Part model, mm, in its own coordinate system. A direction names the side the tool comes from. Give positions to 0.01 mm unless a question says otherwise; leave off trailing zeros. Write each loop counter-clockwise with the first axis right and the second up, starting at its lowest first coordinate (ties: lowest second). Pieces come first, ordered by that corner, then holes. Notation, with made-up numbers: M 64,71.5 L 89,71.5 A28 ccw 89,108.5 Z; hole C 89,27 d9. An arc over 180 degrees is marked long. Answer as CSV lines item,"result". Start each with the question number.
Item 1: Band-saw the part on A-A, the plane z = -46. List the corners of the cut face in (x, y).
Item 2: Wall check: L1, parallel to X at y = 5, z = -35; L2, parallel to X at y = 1.5, z = -44; L3, parallel to X at y = 2.5, z = 23.5. Give the ranges that are in metal, low to high. Write a range as from..to.
Item 3: Two-plate mould, pull along Y, no slides. Class faces 4 (the flat face through (9, 0.9, 64)), 5 (the flat face through (0, 10, 10)), 6 (the flat face through (0, 2, 59)), 7 (the flat face through (20.5, 6, 28)): +Y half, -Y half, draft (parallel to the pull), parting line (faces both ways), or undercut.
Item 4: 3-axis set-ups, long thin cutter, end or side, ignore diameter. For faces 1 (the flat face through (-26, 5, 35)), 2 (the flat face through (12.5, 5, 31)), 3 (the flat face through (-20.5, 6, 28)): which of +Z, -Z, +X, -X, +Y, -Y reach the whole face in a straight line?
Item 5: Pin check, flat tips, straight feed: pin 1 (4 mm diameter, centred on x = -16, z = 18, fed in from +Y); pin 2 (5 mm diameter, centred on y = 3.5, z = -34, fed in from +X); pin 3 (1.2 mm diameter, centred on x = -0.5, y = 1, fed in from +Z); pin 4 (5 mm diameter, centred on x = 25.5, y = 5, fed in from +Z). Stop position of each tip, or through.
Item 6: Band-saw the part on D-D, the plane z = 18. List the corners of the cut face in (x, y).
Item 7: Band-saw the part on C-C, the plane z = 30.5. List the corners of the cut face in (x, y), then the cut area to 3 significant figures.
Item 8: Band-saw the part on B-B, the plane x = -6. List the corners of the cut face in (y, z).
from build123d import *
from OCP.BRepFilletAPI import BRepFilletAPI_MakeChamfer

# Parameters (mm, degrees)
SKETCH1_W               = 24
SKETCH1_H               = 40
BOSS_EXTRUDE1_DEPTH     = 10
SKETCH2_R               = 7.5
BOSS_EXTRUDE2_DEPTH     = 10
SKETCH4_W               = 2
SKETCH4_H               = 20
SKETCH4_H_2             = 16
CUT_EXTRUDE1_DEPTH      = 20
SKETCH5_R               = 2.4
CUT_EXTRUDE2_DEPTH      = 74
CHAMFER3_SIZE           = 2
CHAMFER3_SIZE2          = 4.613601474
BOSS_EXTRUDE3_DEPTH     = 10
CUT_EXTRUDE3_DEPTH      = 10
CUT_EXTRUDE3_DEPTH_BACK = 10
FILLET1_R               = 10
SKETCH8_W               = 5
SKETCH8_H               = 3
CUT_EXTRUDE4_DEPTH      = 5


with BuildPart() as part:
    # Sketch1 → Boss-Extrude1 (new body)
    with BuildSketch(Plane(origin=(0, 0, 0), x_dir=(1, 0, 0), z_dir=(0, 1, 0))):
        Rectangle(SKETCH1_W, SKETCH1_H)
    extrude(amount=BOSS_EXTRUDE1_DEPTH)

    # Sketch2 → Boss-Extrude2 (add)
    with BuildSketch(Plane.XZ):
        Polygon((7, -20), (-7, -20), (-7, 35), (-32, 35), (-32, -15), (-12.5, -25), (-12.5, -50), (12.5, -50), (12.5, -25), (32, -15), (32, 35), (7, 35), align=None)
        with Locations(Location((0, -35, 0), (0, 0, 270))):
            Circle(SKETCH2_R, mode=Mode.SUBTRACT)
        with Locations(Location((-19.5, 18, 0), (0, 0, 270))):
            Circle(SKETCH2_R, mode=Mode.SUBTRACT)
        with Locations(Location((19.5, 18, 0), (0, 0, 270))):
            Circle(SKETCH2_R, mode=Mode.SUBTRACT)
    extrude(amount=-BOSS_EXTRUDE2_DEPTH)

    # Sketch4 → Cut-Extrude1 (cut)
    with BuildSketch(Plane(origin=(0, 10, 0), x_dir=(1, 0, 0), z_dir=(0, 1, 0))):
        with Locations((19.5, -35)):
            Rectangle(SKETCH4_W, SKETCH4_H)
        with Locations((-19.5, -35)):
            Rectangle(SKETCH4_W, SKETCH4_H)
        with Locations((0, 50)):
            Rectangle(SKETCH4_W, SKETCH4_H_2)
    extrude(amount=-CUT_EXTRUDE1_DEPTH, mode=Mode.SUBTRACT)

    # Sketch5 → Cut-Extrude2 (cut)
    with BuildSketch(Plane(origin=(32, 0, 0), x_dir=(0, 0, -1), z_dir=(1, 0, 0))):
        with Locations(Location((-30.5, 5, 0), (0, 0, 180))):
            Circle(SKETCH5_R)
        with Locations(Location((46, 5, 0), (0, 0, 180))):
            Circle(SKETCH5_R)
    extrude(amount=-CUT_EXTRUDE2_DEPTH, mode=Mode.SUBTRACT)

    # Chamfer3: one chamfer whose edges measure the first distance from different faces: ONE call of the kernel's chamfer builder (chamfer() names one face for all edges)
    chamfer3_edges_1 = [part.edges().sort_by_distance(p)[0] for p in [
        (-12.5, 5, -25),
        (-32, 5, -15),
    ]]
    chamfer3_side_1 = [part.faces().sort_by_distance(p)[0] for p in [
        (-22.25, 5, -20),
    ]]
    chamfer3_edges_2 = [part.edges().sort_by_distance(p)[0] for p in [
        (32, 5, -15),
        (12.5, 5, -25),
    ]]
    chamfer3_side_2 = [part.faces().sort_by_distance(p)[0] for p in [
        (22.25, 5, -20),
    ]]
    chamfer3 = BRepFilletAPI_MakeChamfer(part.part.solid().wrapped)
    for e in chamfer3_edges_1:
        chamfer3.Add(CHAMFER3_SIZE, CHAMFER3_SIZE2, e.wrapped, chamfer3_side_1[0].wrapped)  # the first distance lies on this face
    for e in chamfer3_edges_2:
        chamfer3.Add(CHAMFER3_SIZE, CHAMFER3_SIZE2, e.wrapped, chamfer3_side_2[0].wrapped)  # the first distance lies on this face
    add(Compound.cast(chamfer3.Shape()), mode=Mode.REPLACE)

    # Sketch6 → Boss-Extrude3 (add)
    with BuildSketch(Plane.XZ):
        Polygon((-12.5, 22.639119403), (-12.5, 69), (12.5, 69), (12.5, 22.639119403), (7, 20), (-7, 20), align=None)
    extrude(amount=-BOSS_EXTRUDE3_DEPTH)

    # Sketch7 → Cut-Extrude3 (cut, two sides: drawn at the far end of the back side and taken through both)
    with BuildSketch(Plane.XY.offset(69).offset(-CUT_EXTRUDE3_DEPTH_BACK)):
        Polygon((-10.05, 0.9), (-7.5, 0.9), (-7.5, -1.2), (7.5, -1.2), (7.5, 0.9), (10.05, 0.9), (10.05, 3), (-10.05, 3), align=None)
    extrude(amount=CUT_EXTRUDE3_DEPTH + CUT_EXTRUDE3_DEPTH_BACK, mode=Mode.SUBTRACT)

    # Fillet1
    # the kernel refuses this fillet: 10 mm, written as the material it adds along each edge
    with BuildSketch(Plane(origin=(12.5, 0, -29.613601474), x_dir=(0.3065313660894553, 0, 0.9518605578567336), z_dir=(0, 1, 0)), Plane(origin=(-12.5, 0, -29.613601474), x_dir=(0, 0, -1), z_dir=(0, 1, 0))) as fillet1_piece_1:
        with BuildLine():
            CenterArc((FILLET1_R * 0.15704572996, FILLET1_R), FILLET1_R, 252.149681698, 17.850318302)
            Line((-FILLET1_R * 0.149485636129, FILLET1_R * 0.0481394421433), (0, 0))
            Line((0, 0), (FILLET1_R * 0.15704572996, 0))
        make_face()
    extrude(amount=10)
    with BuildSketch(Plane(origin=(14.279634926, 0, -24.087366705), x_dir=(0.8898174628127374, 0, 0.4563166475962744), z_dir=(0, 1, 0)), Plane(origin=(-14.279634926, 0, -24.087366705), x_dir=(0.30653136608945597, 0, -0.9518605578567335), z_dir=(0, 1, 0))) as fillet1_piece_2:
        with BuildLine():
            CenterArc((FILLET1_R * 0.414213562373, FILLET1_R), FILLET1_R, 225, 45)
            Line((-FILLET1_R * 0.292893218813, FILLET1_R * 0.292893218813), (0, 0))
            Line((0, 0), (FILLET1_R * 0.414213562373, 0))
        make_face()
    extrude(amount=10)
    with BuildSketch(Plane(origin=(12.5, 10, 35), x_dir=(0, 0, 1), z_dir=(0, -1, 0))) as fillet1_piece_3:
        with BuildLine():
            CenterArc((9.16515139, -10), FILLET1_R, 90, 66.421821522)
            Line((0, -6), (0, 0))
            Line((0, 0), (9.16515139, 0))
        make_face()
    extrude(amount=10)
    with BuildSketch(Plane(origin=(-12.5, 0, 35), x_dir=(-1, 0, 0), z_dir=(0, 1, 0))) as fillet1_piece_4:
        with BuildLine():
            CenterArc((10, 9.16515139), FILLET1_R, 180, 66.421821522)
            Line((0, 9.16515139), (0, 0))
            Line((0, 0), (6, 0))
        make_face()
    extrude(amount=10)
    # the kernel refuses this fillet: 10 mm, written as the material it takes off along each edge
    with BuildSketch(Plane(origin=(30.220365074, -10.355339059, -15.912633295), x_dir=(-0.8898174628127375, 0, -0.45631664759627466), z_dir=(0, 1, 0))) as fillet1_2_piece_1:
        with BuildLine():
            CenterArc((FILLET1_R * 0.414213562373, FILLET1_R), FILLET1_R, 225, 45)
            Line((-FILLET1_R * 0.292893218813, FILLET1_R * 0.292893218813), (0, 0))
            Line((0, 0), (FILLET1_R * 0.414213562373, 0))
        make_face()
    extrude(amount=30.710678119, mode=Mode.SUBTRACT)
    with BuildSketch(Plane(origin=(32, -3.926143249, -10.386398526), x_dir=(0, 0, 1), z_dir=(0, 1, 0)), Plane(origin=(-32, -3.926143249, -10.386398526), x_dir=(0.3065313660894543, 0, -0.9518605578567341), z_dir=(0, 1, 0))) as fillet1_2_piece_2:
        with BuildLine():
            CenterArc((FILLET1_R * 0.15704572996, -FILLET1_R), FILLET1_R, 90, 17.850318302)
            Line((-FILLET1_R * 0.149485636129, -FILLET1_R * 0.0481394421433), (0, 0))
            Line((0, 0), (FILLET1_R * 0.15704572996, 0))
        make_face()
    extrude(amount=17.852286498, mode=Mode.SUBTRACT)
    with BuildSketch(Plane(origin=(-30.220365074, -10.355339059, -15.912633295), x_dir=(0.889817462812737, 0, -0.45631664759627527), z_dir=(0, 1, 0))) as fillet1_2_piece_3:
        with BuildLine():
            CenterArc((FILLET1_R * 0.414213562373, -FILLET1_R), FILLET1_R, 90, 45)
            Line((-FILLET1_R * 0.292893218813, -FILLET1_R * 0.292893218813), (0, 0))
            Line((0, 0), (FILLET1_R * 0.414213562373, 0))
        make_face()
    extrude(amount=30.710678119, mode=Mode.SUBTRACT)

    # Sketch8 → Cut-Extrude4 (cut)
    with BuildSketch(Plane.XY.offset(59)):
        Rectangle(SKETCH8_W, SKETCH8_H)
    extrude(amount=-CUT_EXTRUDE4_DEPTH, mode=Mode.SUBTRACT)


solid = part.part
Output:
1,outline,"M -12.5,0 L -1,0 L -1,2.6 L -12.5,2.6 Z; M -12.5,7.4 L -1,7.4 L -1,10 L -12.5,10 Z; M 1,0 L 12.5,0 L 12.5,2.6 L 1,2.6 Z; M 1,7.4 L 12.5,7.4 L 12.5,10 L 1,10 Z"
2,L1,"-12.5..-7.5, 7.5..12.5"
2,L2,"-12.5..-1, 1..12.5"
2,L3,"-32..-24.6, -14.4..14.4, 24.6..32"
3,face 4,"undercut"
3,face 5,"+Y half"
3,face 6,"undercut"
3,face 7,"draft"
4,face 1,"+Z, -X, +Y, -Y"
4,face 2,"+X"
4,face 3,"+Z, +Y, -Y"
5,pin 1,"through"
5,pin 2,"x = 12.5"
5,pin 3,"z = 59"
5,pin 4,"z = 35"
6,outline,"M -32,0 L -27,0 L -27,10 L -32,10 Z; M -12,0 L 12,0 L 12,10 L -12,10 Z; M 27,0 L 32,0 L 32,10 L 27,10 Z"
7,outline,"M -32,0 L -20.5,0 L -20.5,2.6 L -32,2.6 Z; M -32,7.4 L -20.5,7.4 L -20.5,10 L -32,10 Z; M -18.5,0 L 18.5,0 L 18.5,2.6 L 12.5,2.6 L 12.5,7.4 L 18.5,7.4 L 18.5,10 L -18.5,10 L -18.5,7.4 L -12.5,7.4 L -12.5,2.6 L -18.5,2.6 Z; M 20.5,0 L 32,0 L 32,2.6 L 20.5,2.6 Z; M 20.5,7.4 L 32,7.4 L 32,10 L 20.5,10 Z"
7,area,"432 mm²"
8,outline,"M 0,-50 L 10,-50 L 10,-39.5 L 0,-39.5 Z; M 0,-30.5 L 10,-30.5 L 10,69 L 3,69 L 3,59 L 0,59 Z; hole C 5,-46 d4.8"
